Verification items for the finished model (mm, model axes). Face numbers are marked on the shaded views. Round coordinates to 2 decimals unless told otherwise and drop trailing zeros. Loops run counter-clockwise (first coordinate to the right, second up) from the corner with the lowest first, then second, coordinate; pieces in that order, holes last. Notation, with made-up numbers: M 5,-28 L 62,-28 A25 ccw 62,6 Z; hole C 80,-30.75 d9. An arc over 180 degrees is marked long. Answer as CSV lines item,"result".
```python
from build123d import *

# Parameters (mm, degrees)
SKETCH1_R           = 253
BOSS_EXTRUDE1_DEPTH = 400
SKETCH2_R           = 210
BOSS_EXTRUDE2_DEPTH = 250
SHELL1_T            = -3
FILLET1_R           = 10


with BuildPart() as part:
    # Sketch1 → Boss-Extrude1 (new body)
    with BuildSketch(Plane.XY):
        Circle(SKETCH1_R)
    extrude(amount=BOSS_EXTRUDE1_DEPTH)

    # Sketch2 → Boss-Extrude2 (add)
    with BuildSketch(Plane.XY.offset(400)):
        Circle(SKETCH2_R)
    extrude(amount=BOSS_EXTRUDE2_DEPTH)

    # Shell1
    shell1_openings = [part.faces().sort_by_distance(p)[0] for p in [
        (0, 0, 0),
        (0, 0, 650),
    ]]
    offset(amount=SHELL1_T, openings=shell1_openings, kind=Kind.INTERSECTION)

    # Fillet1
    # the kernel refuses this fillet: 10 mm, written as the material it adds along each edge
    with BuildSketch(Plane(origin=(0, 0, 400), x_dir=(1, 0, 0), z_dir=(0, -1, 0))) as fillet1_piece_1:
        with BuildLine():
            CenterArc((210 + FILLET1_R, FILLET1_R), FILLET1_R, 180, 90)
            Line((210, FILLET1_R), (210, 0))
            Line((210, 0), (210 + FILLET1_R, 0))
        make_face()
    revolve(axis=Axis((0, 0, 400), (0, 0, 1)))
    # the kernel refuses this fillet: 10 mm, written as the material it takes off along each edge
    with BuildSketch(Plane(origin=(0, 0, 0), x_dir=(1, 0, 0), z_dir=(0, -1, 0))) as fillet1_2_piece_1:
        with BuildLine():
            CenterArc((243, 7.141428429), FILLET1_R, 314.427004001, 45.572995999)
            Line((250, 0), (253, 0))
            Line((253, 0), (253, 7.141428429))
        make_face()
    revolve(axis=Axis((0, 0, 0), (0, 0, 1)), mode=Mode.SUBTRACT)
    with BuildSketch(Plane(origin=(0, 0, 650), x_dir=(1, 0, 0), z_dir=(0, -1, 0))) as fillet1_2_piece_2:
        with BuildLine():
            CenterArc((200, -7.141428429), FILLET1_R, 0, 45.572995999)
            Line((207, 0), (210, 0))
            Line((210, 0), (210, -7.141428429))
        make_face()
    revolve(axis=Axis((0, 0, 650), (0, 0, 1)), mode=Mode.SUBTRACT)


solid = part.part
```
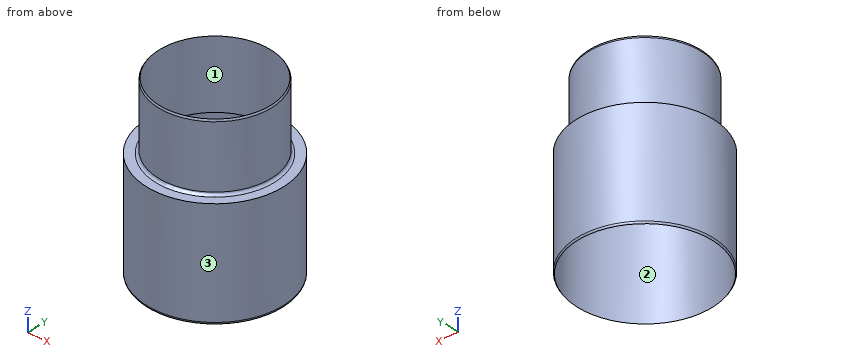
1) Go/stop test with flat-tipped pins: pin 1 (10 mm diameter, centred on x = 53.5, z = 123, fed in from +Y); pin 2 (10 mm diameter, centred on y = 177, z = 262.5, fed in from +X); pin 3 (8 mm diameter, centred on y = -146.5, z = 508, fed in from -X); pin 4 (12 mm diameter, centred on x = -199.5, y = 72.5, fed in from +Z). Record where each tip stops, or that it passes through.
Here are the results:
pin 1,"stops at y = 248.31"
pin 2,"stops at x = 185.54"
pin 3,"stops at x = -154.25"
pin 4,"stops at z = 650"
2) Material ranges on probe 1 along Y at (x, z) = (0, 450); probe 2 along Y at (x, z) = (0, 252); probe 3 along X at (y, z) = (112, 453.5), recorded low to high.
Here are the results:
probe 1,"y = -210 to -207, 207 to 210"
probe 2,"y = -253 to -250, 250 to 253"
probe 3,"x = -177.64 to -174.08, 174.08 to 177.64"
3) Section check A-A (y = 0). Record the cut outline in (x, z), plus the area to 3 significant figures.
Here are the results:
outline,"M -253,7.14 A10 ccw -250,0 L -250,397 L -207,397 L -207,650 A10 ccw -210,642.86 L -210,410 A10 cw -220,400 L -253,400 Z; M 207,397 L 250,397 L 250,0 A10 ccw 253,7.14 L 253,400 L 220,400 A10 cw 210,410 L 210,642.86 A10 ccw 207,650 Z"
area,"4,170 mm^2"
4) Section check C-C (z = 371). Record the cut outline in (x, y), plus the area to 3 significant figures.
Here are the results:
outline,"C 0,0 d506; hole C 0,0 d500"
area,"4,740 mm^2"
5) Section check D-D (z = 585.5). Record the cut outline in (x, y).
Here are the results:
outline,"C 0,0 d420; hole C 0,0 d414"
6) Draft check along X on the marked faces 1, 2 and 3. Enter one of: +X half, -X half, draft (parallel to the pull), parting line (faces both ways), or undercut.
Here are the results:
face 1,"undercut"
face 2,"undercut"
face 3,"parting line"
